Could you check a few things on this drawing? It's one solid part, dimensions in mm from its lowest x, y, z. A direction names the side the tool comes from. Give positions to 0.01 mm unless a question says otherwise; leave off trailing zeros. Order: outer loops, then holes, each group sorted by start corner. A loop starts at its lowest first (then second) coordinate and runs counter-clockwise, first axis right, second up.
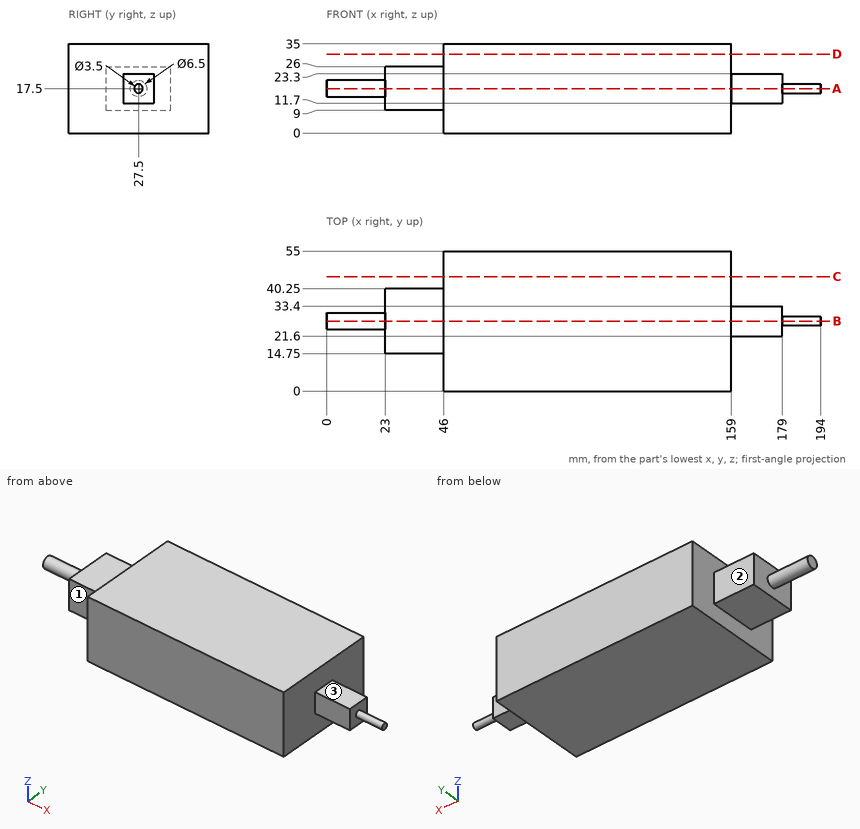
Q1. If we section it at B-B on y = 27.5: List the corners of the cut face in (x, z) for me.
Filled sheet:
outline: (0, 14.25) - (23, 14.25) - (23, 9) - (46, 9) - (46, 0) - (159, 0) - (159, 11.7) - (179, 11.7) - (179, 15.75) - (194, 15.75) - (194, 19.25) - (179, 19.25) - (179, 23.3) - (159, 23.3) - (159, 35) - (46, 35) - (46, 26) - (23, 26) - (23, 20.75) - (0, 20.75) - close
Q2. If we section it at C-C on y = 45: List the corners of the cut face in (x, z) for me, plus the area to 4 significant figures.
Filled sheet:
outline: (46, 0) - (159, 0) - (159, 35) - (46, 35) - close
area: 3,955 mm2
Q3. If we section it at D-D on z = 31: List the corners of the cut face in (x, y) for me, plus the area to 4 significant figures.
Filled sheet:
outline: (46, 0) - (159, 0) - (159, 55) - (46, 55) - close
area: 6,215 mm2
Q4. I need wall thicknesses on L1, parallel to X at y = 13.5, z = 21; L2, parallel to X at y = 16, z = 19.5; L3, parallel to Z at x = 163, y = 22. Which ranges of each line are inside material? Lowest first, please.
Filled sheet:
L1: x = 46 to 159
L2: x = 23 to 159
L3: z = 11.7 to 23.3
Q5. I'm going to push flat-ended pins straight in: P1, Ø3.5, axis at x = 173.5, z = 18, coming from the -Y side; P2, Ø9.5, axis at x = 171.5, y = 27.5, coming from the +Z side; P3, Ø9.5, axis at x = 174, z = 16.5, coming from the +Y side. Where does each tip first touch, or does it pass through?
Filled sheet:
P1: stops at y = 21.6
P2: stops at z = 23.3
P3: stops at y = 33.4
Q6. For the marked faces 1, 2 and 3, which set-ups out of +Z, -Z, +X, -X, +Y, -Y let a thin tool reach every point of the face, with its end or its side?
Filled sheet:
face 1: +Z, -Z, -X, -Y
face 2: +Z, -Z, -X, +Y
face 3: +Z, +X, +Y, -Y
Q7. If we section it at A-A on z = 17.5: List the corners of the cut face in (x, y) for me, plus the area to 3 significant figures.
Filled sheet:
outline: (0, 24.25) - (23, 24.25) - (23, 14.75) - (46, 14.75) - (46, 0) - (159, 0) - (159, 21.6) - (179, 21.6) - (179, 25.75) - (194, 25.75) - (194, 29.25) - (179, 29.25) - (179, 33.4) - (159, 33.4) - (159, 55) - (46, 55) - (46, 40.25) - (23, 40.25) - (23, 30.75) - (0, 30.75) - close
area: 7,240 mm2
